```python
from build123d import *

# Parameters (mm, degrees)
F0_R     = 3.4
F1_DEPTH = 350


with BuildPart() as f1:
    # F0 (on Front) → F1 (new body)
    with BuildSketch(Plane.XZ):
        with BuildLine():
            Line((-67.97487, 38.591727), (-60.67487, 38.591727))
            ThreePointArc((-60.67487, 38.591727), (-58.907103, 39.32396), (-58.17487, 41.091727))
            Line((-58.17487, 41.091727), (-58.17487, 48.391727))
            Line((-58.17487, 48.391727), (-58.97487, 48.391727))
            ThreePointArc((-58.97487, 48.391727), (-59.116292, 48.450306), (-59.17487, 48.591727))
            Line((-59.17487, 48.591727), (-59.17487, 49.491727))
            Line((-59.17487, 49.491727), (-60.37487, 49.491727))
            Line((-60.37487, 49.491727), (-60.37487, 45.341727))
            Line((-60.37487, 45.341727), (-63.369235, 45.341727))
            Line((-63.369235, 45.341727), (-67.37487, 49.347362))
            Line((-67.37487, 49.347362), (-67.37487, 57.836092))
            Line((-67.37487, 57.836092), (-63.369235, 61.841727))
            Line((-63.369235, 61.841727), (-60.37487, 61.841727))
            Line((-60.37487, 61.841727), (-60.37487, 57.691727))
            Line((-60.37487, 57.691727), (-59.17487, 57.691727))
            Line((-59.17487, 57.691727), (-59.17487, 58.591727))
            ThreePointArc((-59.17487, 58.591727), (-59.116292, 58.733149), (-58.97487, 58.791727))
            Line((-58.97487, 58.791727), (-58.17487, 58.791727))
            Line((-58.17487, 58.791727), (-58.17487, 61.841727))
            Line((-58.17487, 61.841727), (-58.17487, 66.091727))
            ThreePointArc((-58.17487, 66.091727), (-58.907103, 67.859494), (-60.67487, 68.591727))
            Line((-60.67487, 68.591727), (-64.92487, 68.591727))
            Line((-64.92487, 68.591727), (-67.97487, 68.591727))
            Line((-67.97487, 68.591727), (-67.97487, 67.891727))
            ThreePointArc((-67.97487, 67.891727), (-68.062738, 67.679595), (-68.27487, 67.591727))
            Line((-68.27487, 67.591727), (-69.07487, 67.591727))
            Line((-69.07487, 67.591727), (-69.07487, 66.391727))
            Line((-69.07487, 66.391727), (-64.92487, 66.391727))
            Line((-64.92487, 66.391727), (-64.92487, 63.397362))
            Line((-64.92487, 63.397362), (-68.930505, 59.391727))
            Line((-68.930505, 59.391727), (-77.419235, 59.391727))
            Line((-77.419235, 59.391727), (-81.42487, 63.397362))
            Line((-81.42487, 63.397362), (-81.42487, 66.391727))
            Line((-81.42487, 66.391727), (-77.27487, 66.391727))
            Line((-77.27487, 66.391727), (-77.27487, 67.591727))
            Line((-77.27487, 67.591727), (-78.07487, 67.591727))
            ThreePointArc((-78.07487, 67.591727), (-78.287002, 67.679595), (-78.37487, 67.891727))
            Line((-78.37487, 67.891727), (-78.37487, 68.591727))
            Line((-78.37487, 68.591727), (-85.67487, 68.591727))
            ThreePointArc((-85.67487, 68.591727), (-87.442637, 67.859494), (-88.17487, 66.091727))
            Line((-88.17487, 66.091727), (-88.17487, 58.791727))
            Line((-88.17487, 58.791727), (-87.37487, 58.791727))
            ThreePointArc((-87.37487, 58.791727), (-87.233449, 58.733149), (-87.17487, 58.591727))
            Line((-87.17487, 58.591727), (-87.17487, 57.691727))
            Line((-87.17487, 57.691727), (-85.97487, 57.691727))
            Line((-85.97487, 57.691727), (-85.97487, 61.841727))
            Line((-85.97487, 61.841727), (-82.980505, 61.841727))
            Line((-82.980505, 61.841727), (-78.97487, 57.836092))
            Line((-78.97487, 57.836092), (-78.97487, 49.347362))
            Line((-78.97487, 49.347362), (-82.980505, 45.341727))
            Line((-82.980505, 45.341727), (-85.97487, 45.341727))
            Line((-85.97487, 45.341727), (-85.97487, 49.491727))
            Line((-85.97487, 49.491727), (-87.17487, 49.491727))
            Line((-87.17487, 49.491727), (-87.17487, 48.591727))
            ThreePointArc((-87.17487, 48.591727), (-87.233449, 48.450306), (-87.37487, 48.391727))
            Line((-87.37487, 48.391727), (-88.17487, 48.391727))
            Line((-88.17487, 48.391727), (-88.17487, 41.091727))
            ThreePointArc((-88.17487, 41.091727), (-87.442637, 39.32396), (-85.67487, 38.591727))
            Line((-85.67487, 38.591727), (-78.37487, 38.591727))
            Line((-78.37487, 38.591727), (-78.37487, 39.291727))
            ThreePointArc((-78.37487, 39.291727), (-78.287002, 39.503859), (-78.07487, 39.591727))
            Line((-78.07487, 39.591727), (-77.27487, 39.591727))
            Line((-77.27487, 39.591727), (-77.27487, 40.791727))
            Line((-77.27487, 40.791727), (-81.42487, 40.791727))
            Line((-81.42487, 40.791727), (-81.42487, 43.786092))
            Line((-81.42487, 43.786092), (-77.419235, 47.791727))
            Line((-77.419235, 47.791727), (-68.930505, 47.791727))
            Line((-68.930505, 47.791727), (-64.92487, 43.786092))
            Line((-64.92487, 43.786092), (-64.92487, 40.791727))
            Line((-64.92487, 40.791727), (-69.07487, 40.791727))
            Line((-69.07487, 40.791727), (-69.07487, 39.591727))
            Line((-69.07487, 39.591727), (-68.27487, 39.591727))
            ThreePointArc((-68.27487, 39.591727), (-68.062738, 39.503859), (-67.97487, 39.291727))
            Line((-67.97487, 39.291727), (-67.97487, 38.591727))
        make_face()
        with BuildLine():
            ThreePointArc((-83.92487, 43.841727), (-83.217764, 43.548834), (-82.92487, 42.841727))
            Line((-82.92487, 42.841727), (-82.92487, 41.091727))
            ThreePointArc((-82.92487, 41.091727), (-83.217764, 40.384621), (-83.92487, 40.091727))
            Line((-83.92487, 40.091727), (-85.67487, 40.091727))
            ThreePointArc((-85.67487, 40.091727), (-86.381977, 40.384621), (-86.67487, 41.091727))
            Line((-86.67487, 41.091727), (-86.67487, 42.841727))
            ThreePointArc((-86.67487, 42.841727), (-86.381977, 43.548834), (-85.67487, 43.841727))
            Line((-85.67487, 43.841727), (-83.92487, 43.841727))
        make_face(mode=Mode.SUBTRACT)
        with BuildLine():
            Line((-62.42487, 43.841727), (-60.67487, 43.841727))
            ThreePointArc((-60.67487, 43.841727), (-59.967764, 43.548834), (-59.67487, 42.841727))
            Line((-59.67487, 42.841727), (-59.67487, 41.091727))
            ThreePointArc((-59.67487, 41.091727), (-59.967764, 40.384621), (-60.67487, 40.091727))
            Line((-60.67487, 40.091727), (-62.42487, 40.091727))
            ThreePointArc((-62.42487, 40.091727), (-63.131977, 40.384621), (-63.42487, 41.091727))
            Line((-63.42487, 41.091727), (-63.42487, 42.841727))
            ThreePointArc((-63.42487, 42.841727), (-63.131977, 43.548834), (-62.42487, 43.841727))
        make_face(mode=Mode.SUBTRACT)
        with BuildLine():
            ThreePointArc((-86.67487, 66.091727), (-86.381977, 66.798834), (-85.67487, 67.091727))
            Line((-85.67487, 67.091727), (-83.92487, 67.091727))
            ThreePointArc((-83.92487, 67.091727), (-83.217764, 66.798834), (-82.92487, 66.091727))
            Line((-82.92487, 66.091727), (-82.92487, 64.341727))
            ThreePointArc((-82.92487, 64.341727), (-83.217764, 63.634621), (-83.92487, 63.341727))
            Line((-83.92487, 63.341727), (-85.67487, 63.341727))
            ThreePointArc((-85.67487, 63.341727), (-86.381977, 63.634621), (-86.67487, 64.341727))
            Line((-86.67487, 64.341727), (-86.67487, 66.091727))
        make_face(mode=Mode.SUBTRACT)
        with Locations((-73.17487, 53.591727)):
            Circle(F0_R, mode=Mode.SUBTRACT)
        with BuildLine():
            ThreePointArc((-59.67487, 64.341727), (-59.967764, 63.634621), (-60.67487, 63.341727))
            Line((-60.67487, 63.341727), (-62.42487, 63.341727))
            ThreePointArc((-62.42487, 63.341727), (-63.131977, 63.634621), (-63.42487, 64.341727))
            Line((-63.42487, 64.341727), (-63.42487, 66.091727))
            ThreePointArc((-63.42487, 66.091727), (-63.131977, 66.798834), (-62.42487, 67.091727))
            Line((-62.42487, 67.091727), (-60.67487, 67.091727))
            ThreePointArc((-60.67487, 67.091727), (-59.967764, 66.798834), (-59.67487, 66.091727))
            Line((-59.67487, 66.091727), (-59.67487, 64.341727))
        make_face(mode=Mode.SUBTRACT)
    extrude(amount=F1_DEPTH)


solid = f1.part
```
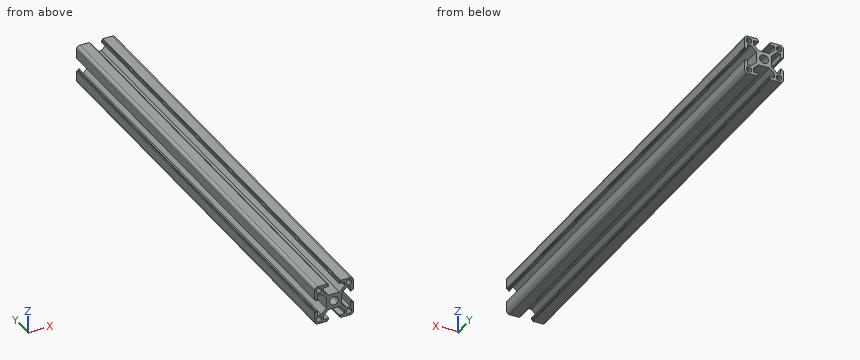
Verification items for the finished model (mm, model axes). Round coordinates to 2 decimals unless told otherwise and drop trailing zeros.
1) Material ranges on line 1 (X direction, y = -314, z = 42); line 2 (Z direction, x = -61, y = -208); line 3 (X direction, y = -106, z = 49), recorded low to high.
Geometry says:
line 1: x = -88.17 to -86.67, -82.92 to -81.42, -64.92 to -63.42, -59.67 to -58.17
line 2: z = 38.59 to 40.09, 43.84 to 45.34, 61.84 to 63.34, 67.09 to 68.59
line 3: x = -87.17 to -85.97, -79.32 to -67.03, -60.37 to -59.17
2) Cross-section at A-A, the plane y = -285. Give the number of separate pieces and of enclosed holes in the cut face, plus the area to 3 significant figures.
Geometry says:
separate pieces: 1
enclosed holes: 5
area: 327 mm2
3) Depth check by flat-ended pin: pin 1 (4 mm diameter, centred on y = -196, z = 56.5, fed in from +X); pin 2 (6 mm diameter, centred on x = -71, z = 52, fed in from +Y); pin 3 (4 mm diameter, centred on x = -75, y = -219, fed in from -Z); pin 4 (1.5 mm diameter, centred on x = -81, z = 55.5, fed in from +Y). Enter the tip coordinate at first touch or a pass-through.
Geometry says:
pin 1: stops at x = -59.17
pin 2: stops at y = 0
pin 3: stops at z = 47.79
pin 4: passes through
